```python
from build123d import *

# Parameters (mm, degrees)
F0_W     = 44
F0_H     = 40
F0_R     = 1.5
F0_R_2   = 5.5
F1_DEPTH = 3.175
F2_W     = 14.666667
F2_H     = 3.175
F3_DEPTH = 3.175


with BuildPart() as f1:
    # F0 (on Front) → F1 (new body)
    with BuildSketch(Plane.XZ):
        Rectangle(F0_W, F0_H)
        with Locations((-12.5, 0)):
            Circle(F0_R, mode=Mode.SUBTRACT)
        Circle(F0_R_2, mode=Mode.SUBTRACT)
        with Locations((12.5, 0)):
            Circle(F0_R, mode=Mode.SUBTRACT)
    extrude(amount=F1_DEPTH)

    # F2 (on face) → F3 (join)
    with BuildSketch(Plane.XY.offset(20)):
        with Locations((-14.666666, -1.5875)):
            Rectangle(F2_W, F2_H)
        with Locations((14.666666, -1.5875)):
            Rectangle(F2_W, F2_H)
    extrude(amount=F3_DEPTH)


solid = f1.part
```
For this review, take the finished solid that the model builds, in its own axes (mm). A direction names the side the tool comes from. Coordinates: 2 decimals unless noted, no trailing zeros. Loops run counter-clockwise (first coordinate to the right, second up) from the corner with the lowest first, then second, coordinate; pieces in that order, holes last. Notation, with made-up numbers: (50.25, 84.5) -> (85.25, 84.5) arc R15 cw to (85.25, 109.5) -> close; hole circle Ø10 at (34.25, -23). An arc over 180 degrees is marked (long way). Return JSON: item names as keys, results as strings. Group by question number.
(1) Consider section D-D, the plane x = 3.5. Give the boundary of the cut face in (y, z) (3 decimals), plus the area to 3 significant figures.
(2) To check wall thickness, follow L1, parallel to Z at x = 12.5, y = -0.8 (3 decimals); L2, parallel to Z at x = 0, y = -1.65; L3, parallel to X at y = -2.65, z = -0.5. State the ranges of each line that lie inside material, in increasing order.
(3) Consider section B-B, the plane x = -12.5. Give the boundary of the cut face in (y, z) (3 decimals), plus the area to 3 significant figures.
(4) For pin 1 Ø1 at (x, y) = (-6, -2.5) entering from +Z, flat-tipped, find the tip position at first contact; note if it passes through.
(5) Tool access review of faces 5 (the flat face through (22, -2, 22)), 6 (the flat face through (7.333, -2, 22)): name each direction out of +Z, -Z, +X, -X, +Y, -Y from which nothing blocks a thin tool from reaching the whole face with its end or side.
(6) Mouldability with a two-part tool opening along Z and no side actions: class faces 1 (the flat face through (0, -2, -20)), 2 (the flat face through (-7.333, -2, 22)), 3 (the cylindrical face through (11, -2, 0)), 4 (the flat face through (-15, -2, 23.175)) as pulls with the +Z half, pulls with the -Z half, needs draft (parallel to the pull), parting line crosses it, or undercut.
(7) Consider section C-C, the plane y = -1.75. Give the boundary of the cut face in (x, z) (3 decimals), plus the area to 3 significant figures.
(8) Consider section A-A, the plane z = 0. Give the boundary of the cut face in (x, y) (3 decimals), plus the area to 3 significant figures.
Results below:
{
 "1": {"outline": "(-3.175, -20) -> (0, -20) -> (0, -4.243) -> (-3.175, -4.243) -> close; (-3.175, 4.243) -> (0, 4.243) -> (0, 20) -> (-3.175, 20) -> close", "area": "100 mm2"},
 "2": {"L1": "z = -20 to -1.5, 1.5 to 23.175", "L2": "z = -20 to -5.5, 5.5 to 20", "L3": "x = -22 to -13.91, -11.09 to -5.48, 5.48 to 11.09, 13.91 to 22"},
 "3": {"outline": "(-3.175, -20) -> (0, -20) -> (0, -1.5) -> (-3.175, -1.5) -> close; (-3.175, 1.5) -> (0, 1.5) -> (0, 23.175) -> (-3.175, 23.175) -> close", "area": "128 mm2"},
 "4": {"pin 1": "stops at z = 20"},
 "5": {"face 5": "+Z, -Z, +X, +Y, -Y", "face 6": "+Z, +Y, -Y"},
 "6": {"face 1": "pulls with the -Z half", "face 2": "needs draft", "face 3": "undercut", "face 4": "pulls with the +Z half"},
 "7": {"outline": "(-22, -20) -> (22, -20) -> (22, 23.175) -> (7.333, 23.175) -> (7.333, 20) -> (-7.333, 20) -> (-7.333, 23.175) -> (-22, 23.175) -> close; hole circle Ø3 at (-12.5, 0); hole circle Ø11 at (0, 0); hole circle Ø3 at (12.5, 0)", "area": "1,740 mm2"},
 "8": {"outline": "(-22, -3.175) -> (-14, -3.175) -> (-14, 0) -> (-22, 0) -> close; (-11, -3.175) -> (-5.5, -3.175) -> (-5.5, 0) -> (-11, 0) -> close; (5.5, -3.175) -> (11, -3.175) -> (11, 0) -> (5.5, 0) -> close; (14, -3.175) -> (22, -3.175) -> (22, 0) -> (14, 0) -> close", "area": "85.7 mm2"}
}
